Work out the finished part from the listing and answer in its coordinate system (mm). A direction names the side the tool comes from. Give positions to 0.01 mm unless a question says otherwise; leave off trailing zeros. Write each loop counter-clockwise with the first axis right and the second up, starting at its lowest first coordinate (ties: lowest second). Pieces come first, ordered by that corner, then holes. Notation, with made-up numbers: (61, 35) -> (84, 35) arc R32 cw to (84, 72) -> close; hole circle Ø11 at (-11, 22). An arc over 180 degrees is marked (long way). Use a Markdown table: item, result. Add a question column.
Q1. Each of these flat-tipped pins is pushed along its axis until it touches: pin 1 Ø1.9 at (x, y) = (122, -44) entering from -Z; pin 2 Ø22.5 at (x, y) = (0, 0) entering from -Z. Where does it stop, or does it pass through?
Q2. Section D-D, the plane z = 34 is taken. Give the vertices of the cut face in (x, y).
Q3. For faces 1 (the face through (94, -44, 3)), 2 (the face through (-0.42, -44.19, -3.68)), 3 (the face through (69, -40.65, 31)), 4 (the face through (27.15, 43.78, 55.64)), 5 (the face through (0, 47, 18)), determine the directions among +Z, -Z, +X, -X, +Y, -Y from which every point of the face is accessible in a straight line to the end or side of a thin tool.
Q4. Consider line 1 (Y direction, x = -21, z = 40.5); line 2 (Y direction, x = 32, z = 37). Determine where each line is inside the solid, lowest interval first.
Q5. For a pull along Y with two mould halves and no side action, classify faces 6 (the face through (0.42, 44.19, -3.68)), 7 (the face through (-27.15, -43.78, 55.64)), 8 (the face through (-14, 1, 0)) as pulls with the +Y half, pulls with the -Y half, needs draft (parallel to the pull), parting line crosses it, or undercut.
Q6. Section A-A, the plane x = 0 is taken. Give the vertices of the cut face in (y, z) (3 decimals), plus the area to 3 significant figures.
Q7. Section B-B, the plane y = 0 is taken. Give the vertices of the cut face in (x, z), plus the area to 3 significant figures.
Q8. Section C-C, the plane z = 5 is taken. Give the vertices of the cut face in (x, y).
from build123d import *

# Parameters (mm, degrees)
SKETCH1_W                      = 60
SKETCH1_H                      = 94
BASE_FLANGE1_DEPTH             = 6.35
EDGE_FLANGE1_STRIP_W           = 31.4
EDGE_FLANGE1_STRIP_H           = 6.35
EDGE_FLANGE1_STRIP_CUT_DEPTH   = 60
EDGE_FLANGE1_STRIP_2_W         = 31.4
EDGE_FLANGE1_STRIP_2_H         = 6.35
EDGE_FLANGE1_STRIP_CUT_2_DEPTH = 60
EDGE_FLANGE1_DEPTH             = 60
EDGE_FLANGE1_BEND_DEPTH        = 60
SKETCH12_W                     = 200
SKETCH12_H                     = 55.65
TAB1_DEPTH                     = 6.35
FILLET2_R                      = 10
SKETCH14_R                     = 12.5
CUT_EXTRUDE1_DEPTH             = 186.873135498
SKETCH15_R                     = 10
CUT_EXTRUDE2_DEPTH             = 203.918265565


# Sheet-metal steps are written as plain solids
with BuildPart() as part:
    # Sketch1 → Base-Flange1 (new body)
    with BuildSketch(Plane.XY):
        Rectangle(SKETCH1_W, SKETCH1_H)
    extrude(amount=-BASE_FLANGE1_DEPTH)

    # Edge-Flange1 strip (across the edge) → Edge-Flange1 strip cut (cut)
    with BuildSketch(Plane(origin=(30, 47, 0), x_dir=(0, -1, 0), z_dir=(-1, 0, 0))):
        with Locations((-6.35, -3.175)):
            Rectangle(EDGE_FLANGE1_STRIP_W, EDGE_FLANGE1_STRIP_H)
    extrude(amount=EDGE_FLANGE1_STRIP_CUT_DEPTH, mode=Mode.SUBTRACT)

    # Edge-Flange1 strip 2 (across the edge) → Edge-Flange1 strip cut 2 (cut)
    with BuildSketch(Plane(origin=(-30, -47, 0), x_dir=(0, 1, 0), z_dir=(1, 0, 0))):
        with Locations((-6.35, -3.175)):
            Rectangle(EDGE_FLANGE1_STRIP_2_W, EDGE_FLANGE1_STRIP_2_H)
    extrude(amount=EDGE_FLANGE1_STRIP_CUT_2_DEPTH, mode=Mode.SUBTRACT)

    # Edge-Flange1 section (across the edge) → Edge-Flange1 (add)
    with BuildSketch(Plane(origin=(30, 47, 0), x_dir=(0, -1, 0), z_dir=(-1, 0, 0))):
        with BuildLine():
            Line((0, 3), (0, 58.65))
            Line((0, 58.65), (6.35, 58.65))
            Line((6.35, 58.65), (6.35, 3))
            ThreePointArc((6.35, 3), (7.228679656, 0.878679656), (9.35, 0))
            Line((9.35, 0), (9.35, -6.35))
            ThreePointArc((9.35, -6.35), (2.738551596, -3.611448404), (0, 3))
        make_face()
    extrude(amount=EDGE_FLANGE1_DEPTH)

    # Edge-Flange1 section 2 (across the edge) → Edge-Flange1 bend (add)
    with BuildSketch(Plane(origin=(-30, -47, 0), x_dir=(0, 1, 0), z_dir=(1, 0, 0))):
        with BuildLine():
            Line((0, 3), (0, 58.65))
            Line((0, 58.65), (6.35, 58.65))
            Line((6.35, 58.65), (6.35, 3))
            ThreePointArc((6.35, 3), (7.228679656, 0.878679656), (9.35, 0))
            Line((9.35, 0), (9.35, -6.35))
            ThreePointArc((9.35, -6.35), (2.738551596, -3.611448404), (0, 3))
        make_face()
    extrude(amount=EDGE_FLANGE1_BEND_DEPTH)

    # Sketch12 → Tab1 (add)
    with BuildSketch(Plane(origin=(0, -40.65, 0), x_dir=(1, 0, 0), z_dir=(0, 1, 0))):
        with Locations((70, -30.825)):
            Rectangle(SKETCH12_W, SKETCH12_H)
    extrude(amount=-TAB1_DEPTH)

    # Fillet2
    fillet2_edges = [part.edges().sort_by_distance(p)[0] for p in [
        (30, 43.825, 58.65),
        (-30, 43.825, 58.65),
        (-30, -43.825, 58.65),
        (170, -43.825, 58.65),
        (170, -43.825, 3),
    ]]
    fillet(fillet2_edges, radius=FILLET2_R)

    # Sketch14 → Cut-Extrude1 (cut, through all)
    with BuildSketch(Plane.XY):
        Circle(SKETCH14_R)
    extrude(amount=-CUT_EXTRUDE1_DEPTH, mode=Mode.SUBTRACT)

    # Sketch15 → Cut-Extrude2 (cut, through all)
    with BuildSketch(Plane(origin=(0, 47, 0), x_dir=(1, 0, 0), z_dir=(0, 1, 0))):
        with Locations(Location((0, -30.825, 0), (0, 0, 270))):
            Circle(SKETCH15_R)
    extrude(amount=-CUT_EXTRUDE2_DEPTH, mode=Mode.SUBTRACT)


solid = part.part
Result set:
| question | item | result |
|---|---|---|
| 1 | pin 1 | stops at z = 3 |
| 1 | pin 2 | passes through |
| 2 | outline | (-30, -47) -> (-9.48, -47) -> (-9.48, -40.65) -> (-30, -40.65) -> close; (-30, 40.65) -> (-9.48, 40.65) -> (-9.48, 47) -> (-30, 47) -> close; (9.48, -47) -> (170, -47) -> (170, -40.65) -> (9.48, -40.65) -> close; (9.48, 40.65) -> (30, 40.65) -> (30, 47) -> (9.48, 47) -> close |
| 3 | face 1 | -Z, +X, +Y, -Y |
| 3 | face 2 | -Z, +X, -X, -Y |
| 3 | face 3 | +Z, +X, -X |
| 3 | face 4 | +Z, +X, +Y |
| 3 | face 5 | +Z, -Z, +X, -X, +Y |
| 4 | line 1 | y = -47 to -40.65, 40.65 to 47 |
| 4 | line 2 | y = -47 to -40.65 |
| 5 | face 6 | pulls with the +Y half |
| 5 | face 7 | needs draft |
| 5 | face 8 | undercut |
| 6 | outline | (-47, 3) arc R9.35 ccw to (-37.65, -6.35) -> (-12.5, -6.35) -> (-12.5, 0) -> (-37.65, 0) arc R3 cw to (-40.65, 3) -> (-40.65, 20.825) -> (-47, 20.825) -> close; (-47, 40.825) -> (-40.65, 40.825) -> (-40.65, 58.65) -> (-47, 58.65) -> close; (12.5, -6.35) -> (37.65, -6.35) arc R9.35 ccw to (47, 3) -> (47, 20.825) -> (40.65, 20.825) -> (40.65, 3) arc R3 cw to (37.65, 0) -> (12.5, 0) -> close; (40.65, 40.825) -> (47, 40.825) -> (47, 58.65) -> (40.65, 58.65) -> close |
| 6 | area | 895 mm2 |
| 7 | outline | (-30, -6.35) -> (-12.5, -6.35) -> (-12.5, 0) -> (-30, 0) -> close; (12.5, -6.35) -> (30, -6.35) -> (30, 0) -> (12.5, 0) -> close |
| 7 | area | 222 mm2 |
| 8 | outline | (-30, -47) -> (166, -47) -> (166, -40.65) -> (-30, -40.65) -> close; (-30, 40.65) -> (30, 40.65) -> (30, 47) -> (-30, 47) -> close |
